from build123d import *

# Parameters (mm, degrees)
F0_W     = 90.9192115068
F0_H     = 16.5890082717
F1_DEPTH = 7.62
F3_R     = 2.5036388288
F4_DEPTH = 10.16
F2_W     = 88.1531853229
F2_H     = 13.1842046976
F5_DEPTH = 7.366


with BuildPart() as f1:
    # F0 (on Top) → F1 (new body)
    with BuildSketch(Plane.XY):
        with Locations((-14.278691262, -52.1163344383)):
            Rectangle(F0_W, F0_H)
    extrude(amount=F1_DEPTH)

    # F3 (on face) → F4 (join)
    with BuildSketch(Plane.XZ.offset(60.4108385742)):
        with Locations((-14.278691262, 4.5239902101)):
            Circle(F3_R)
    extrude(amount=F4_DEPTH)

    # F2 (on face) → F5 (cut)
    with BuildSketch(Plane.XY.offset(7.62)):
        with Locations((-13.8304857537, -51.4442324638)):
            Rectangle(F2_W, F2_H)
    extrude(amount=-F5_DEPTH, mode=Mode.SUBTRACT)


solid = f1.part
Read the model definition and answer for the solid it produces. Units are mm, in the model's axes. A direction names the side the tool comes from. Round coordinates to 2 decimals unless told otherwise and drop trailing zeros. Write each loop counter-clockwise with the first axis right and the second up, starting at its lowest first coordinate (ties: lowest second). Pieces come first, ordered by that corner, then holes. Notation, with made-up numbers: M 51.25,-32 L 93.25,-32 A26 ccw 93.25,-1 Z; hole C 60,-32 d2. An arc over 180 degrees is marked long. Use a Markdown table: item, result.
1) Straight lines are drawn through the part: line 1 along Y through (x, z) = (-8, 4.75); line 2 along X through (y, z) = (-50.5, 1); line 3 along Z through (x, y) = (-1.5, -55.75). For each, find the intervals that lie inside material, in ascending order. Write a range as [from, to].
Answers follow:
| item | result |
|---|---|
| line 1 | y = [-60.41, -58.04], [-44.85, -43.82] |
| line 2 | x = [-59.74, -57.91], [30.25, 31.18] |
| line 3 | z = [0, 0.25] |
2) For a pull along X with two mould halves and no side action, classify faces 4 (the flat face through (-14, -70.571, 5)), 5 (the flat face through (31.181, -52, 4)), 6 (the flat face through (-57.907, -52, 4)) as pulls with the +X half, pulls with the -X half, needs draft (parallel to the pull), parting line crosses it, or undercut.
Answers follow:
| item | result |
|---|---|
| face 4 | needs draft |
| face 5 | pulls with the +X half |
| face 6 | undercut |
3) The part is cut by section B-B (y = -57.25). Write down the section's boundary in (x, z), plus the area to 3 significant figures.
Answers follow:
| item | result |
|---|---|
| outline | M -59.74,0 L 31.18,0 L 31.18,7.62 L 30.25,7.62 L 30.25,0.25 L -57.91,0.25 L -57.91,7.62 L -59.74,7.62 Z |
| area | 43.5 mm2 |
4) Flat-ended cylindrical pins translate along their axes: pin 1 (3.5 mm diameter, centred on x = -8.5, z = 5.5, fed in from -Y); pin 2 (2 mm diameter, centred on y = -63.5, z = 4, fed in from +X); pin 3 (6 mm diameter, centred on x = 13, y = -64, fed in from -Z). Find the tip coordinate at first contact, or state that the pin passes through.
Answers follow:
| item | result |
|---|---|
| pin 1 | stops at y = -60.41 |
| pin 2 | stops at x = -11.78 |
| pin 3 | passes through |
5) The part is cut by section D-D (x = -14). Write down the section's boundary in (y, z).
Answers follow:
| item | result |
|---|---|
| outline | M -70.57,2.04 L -60.41,2.04 L -60.41,0 L -43.82,0 L -43.82,7.62 L -44.85,7.62 L -44.85,0.25 L -58.04,0.25 L -58.04,7.62 L -60.41,7.62 L -60.41,7.01 L -70.57,7.01 Z |
6) The part is cut by section C-C (z = 3.75). Write down the section's boundary in (x, y), plus the area to 3 significant figures.
Answers follow:
| item | result |
|---|---|
| outline | M -59.74,-60.41 L -16.66,-60.41 L -16.66,-70.57 L -11.9,-70.57 L -11.9,-60.41 L 31.18,-60.41 L 31.18,-43.82 L -59.74,-43.82 Z; hole M -57.91,-58.04 L 30.25,-58.04 L 30.25,-44.85 L -57.91,-44.85 Z |
| area | 394 mm2 |
7) A tool of negligible diameter and unlimited length cuts with its end or side. For faces 1 (the cylindrical face through (-11.9, -65.4, 5.3)), 2 (the flat face through (30.246, -52, 4)), 3 (the flat face through (-59.738, -52, 4)), from which of +Z, -Z, +X, -X, +Y, -Y can it reach the whole face along a straight path? Write none if from no direction.
Answers follow:
| item | result |
|---|---|
| face 1 | -Y |
| face 2 | +Z |
| face 3 | +Z, -Z, -X, +Y, -Y |
8) The part is cut by section A-A (x = 16). Write down the section's boundary in (y, z), plus the area to 3 significant figures.
Answers follow:
| item | result |
|---|---|
| outline | M -60.41,0 L -43.82,0 L -43.82,7.62 L -44.85,7.62 L -44.85,0.25 L -58.04,0.25 L -58.04,7.62 L -60.41,7.62 Z |
| area | 29.3 mm2 |
